Verification items for the finished model (mm, model axes). Face numbers are marked on the shaded views. A direction names the side the tool comes from. Round coordinates to 2 decimals unless told otherwise and drop trailing zeros. Write each loop counter-clockwise with the first axis right and the second up, starting at its lowest first coordinate (ties: lowest second). Pieces come first, ordered by that corner, then holes. Notation, with made-up numbers: M 31.5,60.5 L 71.5,60.5 A27 ccw 71.5,93.5 Z; hole C -23,-22 d2. An arc over 180 degrees is marked long. Write each question's results on one line, items separated by ' | '.
from build123d import *

# Parameters (mm, degrees)
F1_DEPTH = 15
F2_R     = 2.063261
F2_R_2   = 2.023213
F3_DEPTH = 1.5


with BuildPart() as f1:
    # F0 (on Front) → F1 (new body)
    with BuildSketch(Plane.XZ):
        Polygon((0, 9.569434), (0, 0), (15.861647, 0), (15.861647, 1.526309), (8.075217, 9.569434), align=None)
    extrude(amount=F1_DEPTH)

    # F2 (on face) → F3 (join)
    with BuildSketch(Plane.XY.offset(9.569434)):
        with Locations((4.037608, -11.90827)):
            Circle(F2_R)
        with Locations((4.037608, -2.994718)):
            Circle(F2_R_2)
    extrude(amount=F3_DEPTH)


solid = f1.part
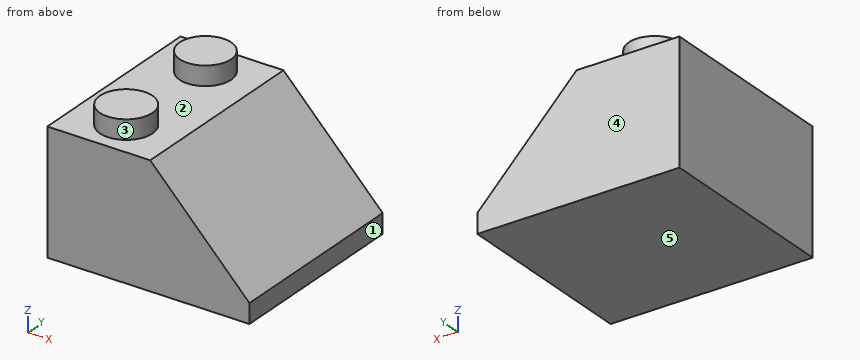
1) Sectioned sample at D-D, the plane z = 2. Record the cut outline in (x, y), and give its area (3 significant figures).
Calculated:
outline: M 0,-15 L 15.4,-15 L 15.4,0 L 0,0 Z | area: 231 mm²
2) Depth check by flat-ended pin: P1, Ø1, axis at y = -1.5, z = 4.5, coming from the +X side. Enter the tip coordinate at first touch or a pass-through.
Calculated:
P1: stops at x = 13.47
3) Sectioned sample at A-A, the plane y = -0.75. Record the cut outline in (x, z), and give its area (3 significant figures).
Calculated:
outline: M 0,0 L 15.86,0 L 15.86,1.53 L 8.08,9.57 L 0,9.57 Z | area: 120 mm²
4) Sectioned sample at B-B, the plane x = 4.5. Record the cut outline in (y, z), and give its area (3 significant figures).
Calculated:
outline: M -15,0 L 0,0 L 0,9.57 L -1.03,9.57 L -1.03,11.07 L -4.96,11.07 L -4.96,9.57 L -9.9,9.57 L -9.9,11.07 L -13.92,11.07 L -13.92,9.57 L -15,9.57 Z | area: 155 mm²
5) Sectioned sample at C-C, the plane z = 10. Record the cut outline in (x, y).
Calculated:
outline: C 4.04,-11.91 d4.13; C 4.04,-2.99 d4.05
6) Access from +Z, -Z, +X, -X, +Y, -Y to the whole of each face (thin tool, end or side, straight path). Record for the marked faces 1 and 2.
Calculated:
face 1: +Z, -Z, +X, +Y, -Y | face 2: +Z
7) Material ranges on line 1 (Z direction, x = 4.5, y = -8); line 2 (X direction, y = -13.5, z = 8.25); line 3 (X direction, y = -10.75, z = 10.5), recorded low to high. Write a range as [from, to].
Calculated:
line 1: z = [0, 9.57] | line 2: x = [0, 9.35] | line 3: x = [2.33, 5.75]
8) Draft check along Y on the marked faces 3, 4 and 5. Enter one of: pulls with the +Y half, pulls with the -Y half, needs draft (parallel to the pull), parting line crosses it, or undercut.
Calculated:
face 3: undercut | face 4: pulls with the +Y half | face 5: needs draft
